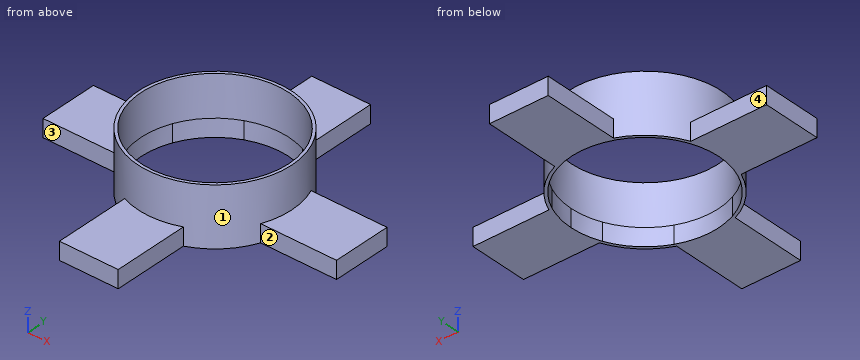
```python
from build123d import *

# Parameters (mm, degrees)
F0_R     = 13.075
F0_R_2   = 12.575
F1_DEPTH = 10
F2_W     = 20
F2_H     = 10
F2_W_2   = 10
F2_H_2   = 20
F3_DEPTH = 3
F4_R     = 12.575
F5_DEPTH = 25


with BuildPart() as f1:
    # F0 (on Top) → F1 (new body)
    with BuildSketch(Plane.XY):
        Circle(F0_R)
        Circle(F0_R_2, mode=Mode.SUBTRACT)
    extrude(amount=F1_DEPTH)

    # F2 (on Top) → F3 (join)
    with BuildSketch(Plane.XY):
        with Locations((15, 0)):
            Rectangle(F2_W, F2_H)
        with Locations((0, -15)):
            Rectangle(F2_W_2, F2_H_2)
        with Locations((-15, 0)):
            Rectangle(F2_W, F2_H)
        with Locations((0, 15)):
            Rectangle(F2_W_2, F2_H_2)
    extrude(amount=F3_DEPTH)

    # F4 (on face) → F5 (cut)
    with BuildSketch(Plane.XY.offset(3)):
        Circle(F4_R)
    extrude(amount=-F5_DEPTH, mode=Mode.SUBTRACT)


solid = f1.part
```
Design review of the part built by this model. Coordinates are the model's own, in mm. Face numbers are marked on the shaded views. A direction names the side the tool comes from. Give positions to 0.01 mm unless a question says otherwise; leave off trailing zeros. Write each loop counter-clockwise with the first axis right and the second up, starting at its lowest first coordinate (ties: lowest second). Pieces come first, ordered by that corner, then holes.
(1) Add section C-C (y = 6). Give the boundary of the cut face in (x, z).
Checked values:
outline: (-11.62, 0) - (-11.05, 0) - (-11.05, 10) - (-11.62, 10) - close; (11.05, 0) - (11.62, 0) - (11.62, 10) - (11.05, 10) - close
(2) Add section A-A (z = 1.75). Give the boundary of the cut face in (x, y) (3 decimals), and give its area (3 significant figures).
Checked values:
outline: (-25, -5) - (-12.081, -5) arc R13.075 ccw to (-5, -12.081) - (-5, -25) - (5, -25) - (5, -12.081) arc R13.075 ccw to (12.081, -5) - (25, -5) - (25, 5) - (12.081, 5) arc R13.075 ccw to (5, 12.081) - (5, 25) - (-5, 25) - (-5, 12.081) arc R13.075 ccw to (-12.081, 5) - (-25, 5) - close; hole circle Ø25.15 at (0, 0)
area: 530 mm2
(3) Tool access review of the marked faces 1, 2, 3 and 4: name each direction out of +Z, -Z, +X, -X, +Y, -Y from which nothing blocks a thin tool from reaching the whole face with its end or side.
Checked values:
face 1: +Z
face 2: +Z, -Z, +X, -Y
face 3: +Z, -Z, -X, -Y
face 4: +Z, -Z, -X, +Y
(4) Clearance check with flat-ended pins moving along their axes: pin 1 Ø1.5 at (x, z) = (13, 1) entering from +Y; pin 2 Ø8 at (x, y) = (17, 5) entering from +Z; pin 3 Ø1.5 at (y, z) = (18.5, 1) entering from -X; pin 4 Ø20 at (x, y) = (0, 0) entering from -Z. State where each tip first meets the part, or that it passes through.
Checked values:
pin 1: stops at y = 5
pin 2: stops at z = 3
pin 3: stops at x = -5
pin 4: passes through
(5) Add section D-D (y = -2.5). Give the boundary of the cut face in (x, z).
Checked values:
outline: (-25, 0) - (-12.32, 0) - (-12.32, 10) - (-12.83, 10) - (-12.83, 3) - (-25, 3) - close; (12.32, 0) - (25, 0) - (25, 3) - (12.83, 3) - (12.83, 10) - (12.32, 10) - close
(6) Add section B-B (x = 0). Give the boundary of the cut face in (y, z) (3 decimals), and give its area (4 significant figures).
Checked values:
outline: (-25, 0) - (-12.575, 0) - (-12.575, 10) - (-13.075, 10) - (-13.075, 3) - (-25, 3) - close; (12.575, 0) - (25, 0) - (25, 3) - (13.075, 3) - (13.075, 10) - (12.575, 10) - close
area: 81.55 mm2
(7) Wall thickness on line 1 along Y through (x, z) = (0, 7) (3 decimals); line 2 along X through (y, z) = (-9, 1): over which ranges is each line inside the solid? List them lowest first.
Checked values:
line 1: y = -13.075 to -12.575, 12.575 to 13.075
line 2: x = -9.48 to -8.78, 8.78 to 9.48
